Source: CAD feature listing. Evaluate the final solid. Frame: model axes, mm. A direction names the side the tool comes from. Give positions to 0.01 mm unless a question says otherwise; leave off trailing zeros. Write each loop counter-clockwise with the first axis right and the second up, starting at its lowest first coordinate (ties: lowest second). Pieces come first, ordered by that corner, then holes.
```python
from build123d import *

# Parameters (mm, degrees)
EXTRUDE_1_DEPTH          = 4
EXTRUDE_2_DEPTH          = 4
SKETCH_3_R               = 5
CUT_EXTRUDE_1_DEPTH      = 4
SKETCH_6_W               = 25
SKETCH_6_H               = 6
CUT_EXTRUDE_4_DEPTH      = 1
CUT_EXTRUDE_4_DEPTH_BACK = 5
SKETCH_7_R               = 2.025
CUT_EXTRUDE_5_DEPTH      = 1
CUT_EXTRUDE_5_DEPTH_BACK = 5
SKETCH_9_R               = 5
EXTRUDE_3_DEPTH          = 4
SKETCH_12_R              = 2.025
CUT_EXTRUDE_8_DEPTH      = 1
CUT_EXTRUDE_8_DEPTH_BACK = 5
CUT_EXTRUDE_9_DEPTH      = 1
CUT_EXTRUDE_9_DEPTH_BACK = 5
EXTRUDE_4_DEPTH          = 4
FILLET_1_R               = 3


with BuildPart() as part:
    # 草图1 → 凸台-拉伸1 (new body)
    with BuildSketch(Plane.XY):
        Polygon((-35, 0), (0, 0), (0, -30), (25, -30), (25, 20), (-35, 20), align=None)
    extrude(amount=EXTRUDE_1_DEPTH)

    # 草图2 → 凸台-拉伸2 (add)
    with BuildSketch(Plane(origin=(0, 0, 0), x_dir=(-1, 0, 0), z_dir=(0, 0, -1))):
        with BuildLine():
            Line((-15.347247215, 38.473341973), (-25, 20))
            Line((-25, 20), (7.6, 20))
            Line((7.6, 20), (-2.052752785, 38.473341973))
            ThreePointArc((-2.052752785, 38.473341973), (-8.7, 42.5), (-15.347247215, 38.473341973))
        make_face()
    extrude(amount=-EXTRUDE_2_DEPTH)

    # 草图3 → 切除-拉伸1 (cut)
    with BuildSketch(Plane(origin=(0, 0, 0), x_dir=(-1, 0, 0), z_dir=(0, 0, -1))):
        with Locations((-8.7, 35)):
            Circle(SKETCH_3_R)
    extrude(amount=-CUT_EXTRUDE_1_DEPTH, mode=Mode.SUBTRACT)

    # 草图6 → 切除-拉伸4 (cut, two sides)
    with BuildSketch(Plane(origin=(0, 0, 0), x_dir=(-1, 0, 0), z_dir=(0, 0, -1))) as cut_extrude_4_sk:
        with Locations((-12.5, -27)):
            Rectangle(SKETCH_6_W, SKETCH_6_H)
    extrude(amount=CUT_EXTRUDE_4_DEPTH, mode=Mode.SUBTRACT)
    extrude(cut_extrude_4_sk.sketch, amount=-CUT_EXTRUDE_4_DEPTH_BACK, mode=Mode.SUBTRACT)

    # 草图7 → 切除-拉伸5 (cut, two sides)
    with BuildSketch(Plane(origin=(0, 0, 0), x_dir=(-1, 0, 0), z_dir=(0, 0, -1))) as cut_extrude_5_sk:
        with Locations((-12.5, -8)):
            Circle(SKETCH_7_R)
        with Locations((-12.5, -18)):
            Circle(SKETCH_7_R)
    extrude(amount=CUT_EXTRUDE_5_DEPTH, mode=Mode.SUBTRACT)
    extrude(cut_extrude_5_sk.sketch, amount=-CUT_EXTRUDE_5_DEPTH_BACK, mode=Mode.SUBTRACT)

    # 草图9 → 凸台-拉伸3 (add)
    with BuildSketch(Plane(origin=(0, 0, 0), x_dir=(-1, 0, 0), z_dir=(0, 0, -1))):
        with BuildLine():
            Line((-20.878399595, 37.817194226), (-25, 20))
            Line((-25, 20), (7.6, 20))
            Line((7.6, 20), (3.478399595, 37.817194226))
            ThreePointArc((3.478399595, 37.817194226), (-8.7, 47.5), (-20.878399595, 37.817194226))
        make_face()
        with Locations((-8.7, 35)):
            Circle(SKETCH_9_R, mode=Mode.SUBTRACT)
    extrude(amount=-EXTRUDE_3_DEPTH)

    # 草图12 → 切除-拉伸8 (cut, two sides)
    with BuildSketch(Plane(origin=(0, 0, 0), x_dir=(-1, 0, 0), z_dir=(0, 0, -1))) as cut_extrude_8_sk:
        with Locations((-15, 10)):
            Circle(SKETCH_12_R)
        with Locations((5, 10)):
            Circle(SKETCH_12_R)
        with Locations((25, 10)):
            Circle(SKETCH_12_R)
    extrude(amount=CUT_EXTRUDE_8_DEPTH, mode=Mode.SUBTRACT)
    extrude(cut_extrude_8_sk.sketch, amount=-CUT_EXTRUDE_8_DEPTH_BACK, mode=Mode.SUBTRACT)

    # 草图13 → 切除-拉伸9 (cut, two sides)
    with BuildSketch(Plane(origin=(0, 0, 0), x_dir=(-1, 0, 0), z_dir=(0, 0, -1))) as cut_extrude_9_sk:
        with BuildLine():
            Line((-25, 20), (7.6, 20))
            Line((7.6, 20), (3.478399595, 37.817194226))
            ThreePointArc((3.478399595, 37.817194226), (-8.7, 47.5), (-20.878399595, 37.817194226))
            Line((-20.878399595, 37.817194226), (-25, 20))
        make_face()
    extrude(amount=CUT_EXTRUDE_9_DEPTH, mode=Mode.SUBTRACT)
    extrude(cut_extrude_9_sk.sketch, amount=-CUT_EXTRUDE_9_DEPTH_BACK, mode=Mode.SUBTRACT)

    # 草图14 → 凸台-拉伸4 (add)
    with BuildSketch(Plane(origin=(0, 0, 0), x_dir=(-1, 0, 0), z_dir=(0, 0, -1))):
        Polygon((0, -6), (6, 0), (0, 0), align=None)
    extrude(amount=-EXTRUDE_4_DEPTH)

    # 圆角1
    fillet_1_edges = [part.edges().sort_by_distance(p)[0] for p in [
        (-35, 20, 2),
        (25, 20, 2),
        (-35, 0, 2),
        (-6, 0, 2),
        (0, -6, 2),
        (25, -24, 2),
        (0, -24, 2),
    ]]
    fillet(fillet_1_edges, radius=FILLET_1_R)


solid = part.part
```
1. Contact query for flat-ended pins moving along their axis: P1, Ø2.5, axis at x = 12.5, y = -18, coming from the +Z side (3 decimals); P2, Ø1.2, axis at y = -13.5, z = 2.5, coming from the -X side; P3, Ø4.5, axis at x = -25, y = 10, coming from the -Z side; P4, Ø1, axis at y = 1.5, z = 2, coming from the -X side. Output: stop coordinate, or through.
2. Cut plane C-C, the plane x = -18.5. Return the cut outline in (y, z), then the cut area to 3 significant figures.
3. Line query: L1, parallel to Y at x = 12.5, z = 2.45 (3 decimals); L2, parallel to Y at x = -31.5, z = 3; L3, parallel to Y at x = -25, z = 1.15 (3 decimals). Output: solid intervals per line, ascending.
4. Cut plane A-A, the plane y = -18. Return the cut outline in (x, z) (3 decimals), then the cut area to 3 significant figures.
5. Cut plane B-B, the plane z = 2.2. Return the cut outline in (x, y) (3 decimals), then the cut area to 3 significant figures.
6. Access query for faces 4 (the flat face through (-20, 0, 2)), 5 (the cylindrical face through (24.14, 19.1, 2.03)). Directions: +Z, -Z, +X, -X, +Y, -Y. A direction counts if a zero-diameter tool reaches every point of the face in a straight line with its end or side. Return the directions, or none.
7. Mould query, pull axis Y, two halves, no side actions, for faces 1 (the cylindrical face through (12.76, -15.99, 1.97)), 2 (the cylindrical face through (-6.079, -0.235, 2.028)), 3 (the flat face through (2, 3, 0)). Classes: +Y half, -Y half, draft (parallel to the pull), parting line (faces both ways), or undercut.
Response values:
1. P1: passes through
1. P2: stops at x = 0
1. P3: stops at z = 0
1. P4: stops at x = -34.83
2. outline: (0, 0) - (20, 0) - (20, 4) - (0, 4) - close
2. area: 80.0 mm2
3. L1: y = -24 to -20.025, -15.975 to -10.025, -5.975 to 20
3. L2: y = 0 to 20
3. L3: y = 0 to 7.975, 12.025 to 20
4. outline: (0, 0) - (10.475, 0) - (10.475, 4) - (0, 4) - close; (14.525, 0) - (25, 0) - (25, 4) - (14.525, 4) - close
4. area: 83.8 mm2
5. outline: (-35, 3) arc R3 ccw to (-32, 0) - (-7.243, 0) arc R3 cw to (-5.121, -0.879) - (-0.879, -5.121) arc R3 cw to (0, -7.243) - (0, -21) arc R3 ccw to (3, -24) - (22, -24) arc R3 ccw to (25, -21) - (25, 17) arc R3 ccw to (22, 20) - (-32, 20) arc R3 ccw to (-35, 17) - close; hole circle Ø4.05 at (-25, 10); hole circle Ø4.05 at (-5, 10); hole circle Ø4.05 at (12.5, -18); hole circle Ø4.05 at (12.5, -8); hole circle Ø4.05 at (15, 10)
5. area: 1,740 mm2
6. face 4: +Z, -Z, -X, -Y
6. face 5: +Z, -Z, +X, +Y
7. face 1: undercut
7. face 2: -Y half
7. face 3: draft
